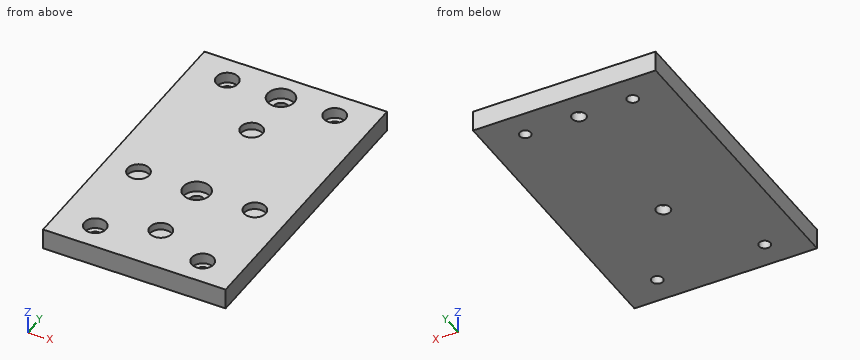
from build123d import *

# Parameters (mm, degrees)
SKETCH1_W           = 68
SKETCH1_H           = 110
SKETCH1_R           = 2.1
SKETCH1_R_2         = 4.05
SKETCH1_R_3         = 2.6
BOSS_EXTRUDE1_DEPTH = 7.7
SKETCH2_R           = 6.304633146
SKETCH2_R_2         = 7.334333348
SKETCH2_R_3         = 8.114040952
SKETCH2_R_4         = 11.073656437
BOSS_EXTRUDE2_DEPTH = 5
SKETCH3_R           = 4.05
SKETCH3_R_2         = 5
CUT_EXTRUDE1_DEPTH  = 4


with BuildPart() as part:
    # Sketch1 → Boss-Extrude1 (new body)
    with BuildSketch(Plane.XY):
        Rectangle(SKETCH1_W, SKETCH1_H)
        with Locations((20, 45)):
            Circle(SKETCH1_R, mode=Mode.SUBTRACT)
        with Locations((-20, 45)):
            Circle(SKETCH1_R, mode=Mode.SUBTRACT)
        with Locations((20, -45)):
            Circle(SKETCH1_R, mode=Mode.SUBTRACT)
        with Locations((-20, -45)):
            Circle(SKETCH1_R, mode=Mode.SUBTRACT)
        with Locations((21.650635095, -12.5)):
            Circle(SKETCH1_R_2, mode=Mode.SUBTRACT)
        with Locations((0, 25)):
            Circle(SKETCH1_R_2, mode=Mode.SUBTRACT)
        with Locations((-21.650635095, -12.5)):
            Circle(SKETCH1_R_2, mode=Mode.SUBTRACT)
        with Locations((0, -36.95)):
            Circle(SKETCH1_R_2, mode=Mode.SUBTRACT)
        with Locations((0, 45)):
            Circle(SKETCH1_R_3, mode=Mode.SUBTRACT)
        with Locations((0, -12.5)):
            Circle(SKETCH1_R_3, mode=Mode.SUBTRACT)
    extrude(amount=BOSS_EXTRUDE1_DEPTH)

    # Sketch2 → Boss-Extrude2 (add)
    with BuildSketch(Plane(origin=(0, 0, 0), x_dir=(-1, 0, 0), z_dir=(0, 0, -1))):
        with Locations((-21.650635095, -12.5)):
            Circle(SKETCH2_R)
        with Locations((0, 25)):
            Circle(SKETCH2_R_2)
        with Locations((21.650635095, -12.5)):
            Circle(SKETCH2_R_3)
        with Locations((0, -36.95)):
            Circle(SKETCH2_R_4)
    extrude(amount=-BOSS_EXTRUDE2_DEPTH)

    # Sketch3 → Cut-Extrude1 (cut)
    with BuildSketch(Plane(origin=(0, 0, 7.7), x_dir=(-1, 0, 0), z_dir=(0, 0, -1))):
        with Locations((-20, 45)):
            Circle(SKETCH3_R)
        with Locations((20, 45)):
            Circle(SKETCH3_R)
        with Locations((-20, -45)):
            Circle(SKETCH3_R)
        with Locations((20, -45)):
            Circle(SKETCH3_R)
        with Locations((0, 45)):
            Circle(SKETCH3_R_2)
        with Locations((0, -12.5)):
            Circle(SKETCH3_R_2)
    extrude(amount=CUT_EXTRUDE1_DEPTH, mode=Mode.SUBTRACT)


solid = part.part
Source: CAD feature listing. Evaluate the final solid. Frame: model axes, mm. Give positions to 0.01 mm unless a question says otherwise; leave off trailing zeros. Order: outer loops, then holes, each group sorted by start corner. A loop starts at its lowest first (then second) coordinate and runs counter-clockwise, first axis right, second up. Notation, with made-up numbers: (-40, -35.75) -> (-13, -35.75) arc R16 ccw to (-13, -12.75) -> close; hole circle Ø1 at (16.5, 33.25). An arc over 180 degrees is marked (long way). Write item = value, one per line.
Item 1: Section query C-C (y = -45). Output: boundary loops of the cut face in (x, z).
Check result:
outline = (-34, 0) -> (-22.1, 0) -> (-22.1, 3.7) -> (-24.05, 3.7) -> (-24.05, 7.7) -> (-34, 7.7) -> close; (-17.9, 0) -> (17.9, 0) -> (17.9, 3.7) -> (15.95, 3.7) -> (15.95, 7.7) -> (-15.95, 7.7) -> (-15.95, 3.7) -> (-17.9, 3.7) -> close; (22.1, 0) -> (34, 0) -> (34, 7.7) -> (24.05, 7.7) -> (24.05, 3.7) -> (22.1, 3.7) -> close
Item 2: Ray query, probe 1 along Y at (x, z) = (0, 6.3); probe 2 along X at (y, z) = (45, 1.7); probe 3 along Y at (x, z) = (-20, 6.35). Return the intervals inside material, ascending.
Check result:
probe_1 = -55 to -41, -32.9 to -17.5, -7.5 to 20.95, 29.05 to 40, 50 to 55
probe_2 = -34 to -22.1, -17.9 to -2.6, 2.6 to 17.9, 22.1 to 34
probe_3 = -55 to -49.05, -40.95 to -16.2, -8.8 to 40.95, 49.05 to 55
Item 3: Section query B-B (x = 0). Output: boundary loops of the cut face in (y, z).
Check result:
outline = (-55, 0) -> (-15.1, 0) -> (-15.1, 3.7) -> (-17.5, 3.7) -> (-17.5, 7.7) -> (-32.9, 7.7) -> (-32.9, 5) -> (-41, 5) -> (-41, 7.7) -> (-55, 7.7) -> close; (-9.9, 0) -> (42.4, 0) -> (42.4, 3.7) -> (40, 3.7) -> (40, 7.7) -> (29.05, 7.7) -> (29.05, 5) -> (20.95, 5) -> (20.95, 7.7) -> (-7.5, 7.7) -> (-7.5, 3.7) -> (-9.9, 3.7) -> close; (47.6, 0) -> (55, 0) -> (55, 7.7) -> (50, 7.7) -> (50, 3.7) -> (47.6, 3.7) -> close
Item 4: Section query D-D (z = 6.5). State how many separate pieces and enclosed holes the cut face has, then the cut area to 3 significant figures.
Check result:
separate_pieces = 1
enclosed_holes = 10
area = 6,910 mm²
Item 5: Section query A-A (y = 45). Output: boundary loops of the cut face in (x, z), then the cut area to 3 significant figures.
Check result:
outline = (-34, 0) -> (-22.1, 0) -> (-22.1, 3.7) -> (-24.05, 3.7) -> (-24.05, 7.7) -> (-34, 7.7) -> close; (-17.9, 0) -> (-2.6, 0) -> (-2.6, 3.7) -> (-5, 3.7) -> (-5, 7.7) -> (-15.95, 7.7) -> (-15.95, 3.7) -> (-17.9, 3.7) -> close; (2.6, 0) -> (17.9, 0) -> (17.9, 3.7) -> (15.95, 3.7) -> (15.95, 7.7) -> (5, 7.7) -> (5, 3.7) -> (2.6, 3.7) -> close; (22.1, 0) -> (34, 0) -> (34, 7.7) -> (24.05, 7.7) -> (24.05, 3.7) -> (22.1, 3.7) -> close
area = 368 mm²
Item 6: Contact query for flat-ended pins moving along their axis: pin 1 (5 mm diameter, centred on x = 20, y = 45, fed in from +Z); pin 2 (1 mm diameter, centred on x = -21.5, y = -9, fed in from +Z). Output: stop coordinate, or through.
Check result:
pin_1 = 3.7
pin_2 = 5
